Autodesk Inventor part; units mm, degrees
ref_plane "Начальная плоскость" through (0, 0, -22.5) normal (0, 0, 1) x (1, 0, 0)
ref_plane "Конечная плоскость" through (0, 0, 692.5) normal (0, 0, 1) x (1, 0, 0)
ref_plane "РабПлоскость4" through (-1.43, 0, -22.5) normal (0.7071, 0, -0.7071) x (-0.7071, 0, -0.7071)
ref_plane "Начальная плоскость" through (0, 0, -22.5) normal (0, 0, 1) x (1, 0, 0)
ref_plane "Конечная плоскость" through (0, 0, 692.5) normal (0, 0, 1) x (1, 0, 0)
sketch "Эскиз" plane through (0, 0, 0) normal (0, 0, 1) x (1, 0, 0)
  line L0 (-1.43, 0) -> (-1.43, 40)
  line L1 (-1.43, 40) -> (43.57, 40)
  line L2 (43.57, 40) -> (43.57, 38.1774)
  line L3 (39.9881, 34.1993) -> (11.2338, 31.1771)
  line L4 (4.07, 23.221) -> (4.07, 0)
  line L5 (4.07, 0) -> (-1.43, 0) construction
  line L6 (23.82, 40) -> (23.82, 32.5) construction
  line L7 (43.57, 34.5758) -> (43.57, 32.5) construction
  line L8 (43.57, 32.5) -> (23.82, 32.5) construction
  line L9 (0, 15) -> (0, -27) construction
  line L10 (-5.539, 0) -> (16.0067, 0) construction
  line L11 (-1.43, 0) -> (-1.43, -40)
  line L12 (-1.43, -40) -> (43.57, -40)
  line L13 (43.57, -40) -> (43.57, -38.1774)
  line L14 (39.9881, -34.1993) -> (11.2338, -31.1771)
  line L15 (4.07, -23.221) -> (4.07, 0)
  arc A0 (11.2338, 31.1771) -> (4.07, 23.221) centre (12.07, 23.221) ccw
  arc A1 (4.07, -23.221) -> (11.2338, -31.1771) centre (12.07, -23.221) ccw
  arc A2 (39.9881, 34.1993) -> (43.57, 38.1774) centre (39.57, 38.1774) ccw
  arc A3 (43.57, -38.1774) -> (39.9881, -34.1993) centre (39.57, -38.1774) ccw
  line L16 (0, 56) -> (0, -56) construction
  line L17 (-15.5135, 0) -> (54.308, 0) construction
  point P0 (4.07, 30.4242)
  point P1 (43.57, -34.5758)
  point P2 (4.07, -30.4242)
  point P3 (23.82, -40)
  point P4 (23.82, -32.5)
  dimension "d0" = 5.5
  dimension "d1" = 40
  dimension "d2" = 45
  dimension "d3" = 7.5
  dimension "d4" = 19.75
  dimension "d5" = 2.0758
  dimension "d23" = 8
  dimension "d24" = 4
  dimension "d25" = 1.43
extrude "Тело" add sketch "Эскиз" along normal up to surface (715 mm away) from surface at -22.5
sketch "Sketch3" plane through (0, 0, 0) normal (0, 0, 1) x (1, 0, 0)
  line L0 (0, 0) -> (10, 0)
ref_plane "Work Plane3" through (0, 0, 0) normal (0, -1, 0) x (1, 0, 0)
sketch "Sketch4" plane through (0, 0, 0) normal (0, -1, 0) x (1, 0, 0)
  line L0 (-2, -22.5) -> (12, -22.5)
  line L1 (-2, 692.5) -> (12, 692.5)
  dimension "d29" = 715
ref_plane "РабПлоскость4" through (-1.43, 0, -22.5) normal (0.7071, 0, -0.7071) x (-0.7071, 0, -0.7071)
split "Разделение1" plane through (-1.43, 0, -22.5) removes the side toward (0.7071, 0, -0.7071)
ref_plane "РабПлоскость5" through (-1.43, 0, 692.5) normal (0.7071, 0, 0.7071) x (0.7071, 0, -0.7071)
split "Разделение2" plane through (-1.43, 0, 692.5) removes the side toward (0.7071, 0, 0.7071)
equation "\"d0\" = G_T"
equation "\"d1\" = 0.5 * G_H"
equation "\"d2\" = G_W"
equation "\"d3\" = G_T1"
equation "\"d4\" = G_C"
equation "\"d23\" = G_IR"
equation "\"d24\" = G_ER"
equation "\"d25\" = ex"
equation "\"d6\" = G_L"
equation "\"G_W\" = 45"
equation "\"G_T\" = 5.5"
equation "\"G_T1\" = 7.5"
equation "\"G_NG\" = 0.105104"
equation "\"G_ER\" = 4"
equation "\"G_IR\" = 8"
equation "\"G_C\" = 19.75"
equation "\"G_L\" = d29"
equation "\"ex\" = 1.43"
equation "\"G_OFFSET_START\" = 22.5"
equation "\"G_OFFSET_END\" = 22.5"
equation "\"d26\" = -G_OFFSET_START"
equation "\"d27\" = G_OFFSET_END + B_L"
properties part number "ISO 657/11 - CH 80 x 8 - 715" material "Сталь, мягкая"
Work out the finished part from the listing and answer in its coordinate system (mm). A direction names the side the tool comes from. Give positions to 0.01 mm unless a question says otherwise; leave off trailing zeros. Write each loop counter-clockwise with the first axis right and the second up, starting at its lowest first coordinate (ties: lowest second). Pieces come first, ordered by that corner, then holes.
(1) A flat-ended cylindrical pin translates along its axis: pin 1 Ø14 at (y, z) = (-10.5, 171.5) entering from +X. Find the tip coordinate at first contact, or state that the pin passes through.
Final values:
pin 1: stops at x = 4.07
(2) Straight lines are drawn through the part: line 1 (Y direction, x = 12, z = 450); line 2 (Y direction, x = 40, z = 336); line 3 (X direction, y = 19, z = 372.5). For each, find the intervals that lie inside material, in ascending order.
Final values:
line 1: y = -40 to -31.26, 31.26 to 40
line 2: y = -40 to -34.2, 34.2 to 40
line 3: x = -1.43 to 4.07
(3) The part is cut by section A-A on x = 27.5. Write down the section's boundary in (y, z).
Final values:
outline: (-40, 6.43) - (-32.89, 6.43) - (-32.89, 663.57) - (-40, 663.57) - close; (32.89, 6.43) - (40, 6.43) - (40, 663.57) - (32.89, 663.57) - close
(4) Which of the six approach directions +Z, -Z, +X, -X, +Y, -Y give full straight-line access (tool end or side, diameter ignored) to faces 1 (the flat face through (-1.43, -1, 330)), 2 (the flat face through (4.07, 0, 330))?
Final values:
face 1: +Z, -Z, -X, +Y, -Y
face 2: +Z, -Z, +X
(5) The mould has two halves that part along Y. Classify faces 3 (the flat face through (2.63, 0.19, -18.44)), 4 (the flat face through (21, -40, 330)), 5 (the flat face through (25.81, 32.71, 330.17)), 6 (the flat face through (21, 40, 330)): pulls with the +Y half, pulls with the -Y half, needs draft (parallel to the pull), parting line crosses it, or undercut.
Final values:
face 3: needs draft
face 4: pulls with the -Y half
face 5: undercut
face 6: pulls with the +Y half
(6) The part is cut by section C-C on y = -9.5. Write down the section's boundary in (x, z), plus the area to 3 significant figures.
Final values:
outline: (-1.43, -22.5) - (4.07, -17) - (4.07, 687) - (-1.43, 692.5) - close
area: 3,900 mm2
(7) The part is cut by section B-B on z = 488. Write down the section's boundary in (x, y).
Final values:
outline: (-1.43, -40) - (43.57, -40) - (43.57, -38.18) arc R4 ccw to (39.99, -34.2) - (11.23, -31.18) arc R8 cw to (4.07, -23.22) - (4.07, 23.22) arc R8 cw to (11.23, 31.18) - (39.99, 34.2) arc R4 ccw to (43.57, 38.18) - (43.57, 40) - (-1.43, 40) - close
